Check sheet for the modelled part. Datum: model origin and axes. Units: mm. A direction names the side the tool comes from. Give positions to 0.01 mm unless a question says otherwise; leave off trailing zeros. Write each loop counter-clockwise with the first axis right and the second up, starting at its lowest first coordinate (ties: lowest second). Pieces come first, ordered by that corner, then holes. Notation, with made-up numbers: M 79.5,83.25 L 83.5,83.25 A34 ccw 83.5,113.25 Z; hole C 10,79 d10. An arc over 180 degrees is marked long. Write item = value, one per line. Start each with the question number.
1) Cross-section at D-D, the plane x = -13.5. Record the cut outline in (y, z) (3 decimals), plus the area to 3 significant figures.
2) Scan lines: line 1 along Z through (x, y) = (-19, 3); line 2 along Y through (x, z) = (-14, 31.5) (3 decimals); line 3 along Y through (x, z) = (-69, 16). Record each from-to range of solid material in increasing order. Write a range as [from, to].
3) Go/stop test with flat-tipped pins: pin 1 (4 mm diameter, centred on x = -35.5, y = -16, fed in from +Z); pin 2 (6 mm diameter, centred on x = -67, z = 0, fed in from -Y); pin 3 (24 mm diameter, centred on x = -53, y = -26, fed in from -Z). Record where each tip stops, or that it passes through.
4) Access from +Z, -Z, +X, -X, +Y, -Y to the whole of each face (thin tool, end or side, straight path). Record for faces 4 (the cylindrical face through (-45.748, 3.131, -4.598)), 5 (the flat face through (-46, 3.175, 40)), 6 (the flat face through (-45, 0.635, 54)).
5) Cross-section at C-C, the plane x = -59. Record the cut outline in (y, z) (3 decimals), plus the area to 3 significant figures.
6) Mould release check, pull along X, two halves, no side actions. Record for faces 1 (the flat face through (-46, -45, 55.608)), 2 (the cylindrical face through (-16.79, 3.13, -4.6)), 3 (the flat face through (-88.382, -17, 25)): released by +X, released by -X, zero draft, split by the parting line, or undercut.
7) Cross-section at B-B, the plane y = 2. Give the number of separate pieces and of enclosed holes in the cut face, plus the area to 3 significant figures.
8) Cross-section at A-A, the plane z = 37. Record the cut outline in (x, y) (3 decimals), plus the area to 3 significant figures.
```python
from build123d import *

# Parameters (mm, degrees)
SKETCH1_W           = 85.09
SKETCH1_H           = 38.1
SKETCH1_R           = 2.38125
BOSS_EXTRUDE1_DEPTH = 6.35
SKETCH2_W           = 85.09
SKETCH2_H           = 6.35
BOSS_EXTRUDE2_DEPTH = 47.625
SKETCH3_W           = 85.09
SKETCH3_H           = 3.175
BOSS_EXTRUDE3_DEPTH = 27.94
SKETCH4_W           = 2.54
SKETCH4_H           = 2.54
BOSS_EXTRUDE4_DEPTH = 85.09


with BuildPart() as part:
    # Sketch1 → Boss-Extrude1 (new body)
    with BuildSketch(Plane(origin=(0, 0, 0), x_dir=(1, 0, 0), z_dir=(0, 1, 0))):
        with Locations((-45.836632653, -8.617857143)):
            Rectangle(SKETCH1_W, SKETCH1_H)
        with Locations(Location((-82.031632653, 4.082142857, 0), (0, 0, 270))):
            Circle(SKETCH1_R, mode=Mode.SUBTRACT)
        with Locations(Location((-77.205632653, 4.082142857, 0), (0, 0, 270))):
            Circle(SKETCH1_R, mode=Mode.SUBTRACT)
        with Locations(Location((-72.379632653, 4.082142857, 0), (0, 0, 270))):
            Circle(SKETCH1_R, mode=Mode.SUBTRACT)
        with Locations(Location((-67.553632653, 4.082142857, 0), (0, 0, 270))):
            Circle(SKETCH1_R, mode=Mode.SUBTRACT)
        with Locations(Location((-62.727632653, 4.082142857, 0), (0, 0, 270))):
            Circle(SKETCH1_R, mode=Mode.SUBTRACT)
        with Locations(Location((-57.901632653, 4.082142857, 0), (0, 0, 270))):
            Circle(SKETCH1_R, mode=Mode.SUBTRACT)
        with Locations(Location((-53.075632653, 4.082142857, 0), (0, 0, 270))):
            Circle(SKETCH1_R, mode=Mode.SUBTRACT)
        with Locations(Location((-48.249632653, 4.082142857, 0), (0, 0, 270))):
            Circle(SKETCH1_R, mode=Mode.SUBTRACT)
        with Locations(Location((-43.423632653, 4.082142857, 0), (0, 0, 270))):
            Circle(SKETCH1_R, mode=Mode.SUBTRACT)
        with Locations(Location((-38.597632653, 4.082142857, 0), (0, 0, 270))):
            Circle(SKETCH1_R, mode=Mode.SUBTRACT)
        with Locations(Location((-33.771632653, 4.082142857, 0), (0, 0, 270))):
            Circle(SKETCH1_R, mode=Mode.SUBTRACT)
        with Locations(Location((-28.945632653, 4.082142857, 0), (0, 0, 270))):
            Circle(SKETCH1_R, mode=Mode.SUBTRACT)
        with Locations(Location((-24.119632653, 4.082142857, 0), (0, 0, 270))):
            Circle(SKETCH1_R, mode=Mode.SUBTRACT)
        with Locations(Location((-19.293632653, 4.082142857, 0), (0, 0, 270))):
            Circle(SKETCH1_R, mode=Mode.SUBTRACT)
        with Locations(Location((-14.467632653, 4.082142857, 0), (0, 0, 270))):
            Circle(SKETCH1_R, mode=Mode.SUBTRACT)
        with Locations(Location((-9.641632653, 4.082142857, 0), (0, 0, 270))):
            Circle(SKETCH1_R, mode=Mode.SUBTRACT)
    extrude(amount=BOSS_EXTRUDE1_DEPTH)

    # Sketch2 → Boss-Extrude2 (add)
    with BuildSketch(Plane.XZ):
        with Locations((-45.836632653, 24.492857143)):
            Rectangle(SKETCH2_W, SKETCH2_H)
    extrude(amount=BOSS_EXTRUDE2_DEPTH)

    # Sketch3 → Boss-Extrude3 (add)
    with BuildSketch(Plane.XY.offset(27.667857143)):
        with Locations((-45.836632653, 4.7625)):
            Rectangle(SKETCH3_W, SKETCH3_H)
        with Locations((-45.836632653, -46.0375)):
            Rectangle(SKETCH3_W, SKETCH3_H)
    extrude(amount=BOSS_EXTRUDE3_DEPTH)

    # Sketch4 → Boss-Extrude4 (add)
    with BuildSketch(Plane(origin=(-3.291632653, 0, 0), x_dir=(0, 0, -1), z_dir=(1, 0, 0))):
        with Locations((-54.337857143, 1.905)):
            Rectangle(SKETCH4_W, SKETCH4_H)
        with Locations((-54.337857143, -43.18)):
            Rectangle(SKETCH4_W, SKETCH4_H)
    extrude(amount=-BOSS_EXTRUDE4_DEPTH)


solid = part.part
```
Reply:
q1.outline = M -47.625,21.318 L 0,21.318 L 0,-1.906 L 6.35,-1.906 L 6.35,55.608 L 0.635,55.608 L 0.635,53.068 L 3.175,53.068 L 3.175,27.668 L -44.45,27.668 L -44.45,53.068 L -41.91,53.068 L -41.91,55.608 L -47.625,55.608 Z; M 0,-10.432 L 6.35,-10.432 L 6.35,-6.258 L 0,-6.258 Z
q1.area = 707 mm2
q2.line_1 = [-10.43, -6.45], [-1.72, 27.67], [53.07, 55.61]
q2.line_2 = [-47.625, -44.45], [3.175, 6.35]
q2.line_3 = [0, 6.35]
q3.pin_1 = 27.67
q3.pin_2 = 0
q3.pin_3 = 21.32
q4.face_4 = +Y, -Y
q4.face_5 = +X, -X
q4.face_6 = +Z, +X, -X
q5.outline = M -47.625,21.318 L 0,21.318 L 0,-1.969 L 6.35,-1.969 L 6.35,55.608 L 0.635,55.608 L 0.635,53.068 L 3.175,53.068 L 3.175,27.668 L -44.45,27.668 L -44.45,53.068 L -41.91,53.068 L -41.91,55.608 L -47.625,55.608 Z; M 0,-10.432 L 6.35,-10.432 L 6.35,-6.195 L 0,-6.195 Z
q5.area = 708 mm2
q6.face_1 = zero draft
q6.face_2 = undercut
q6.face_3 = released by -X
q7.separate_pieces = 2
q7.enclosed_holes = 16
q7.area = 3,170 mm2
q8.outline = M -88.382,-47.625 L -3.292,-47.625 L -3.292,-44.45 L -88.382,-44.45 Z; M -88.382,3.175 L -3.292,3.175 L -3.292,6.35 L -88.382,6.35 Z
q8.area = 540 mm2
